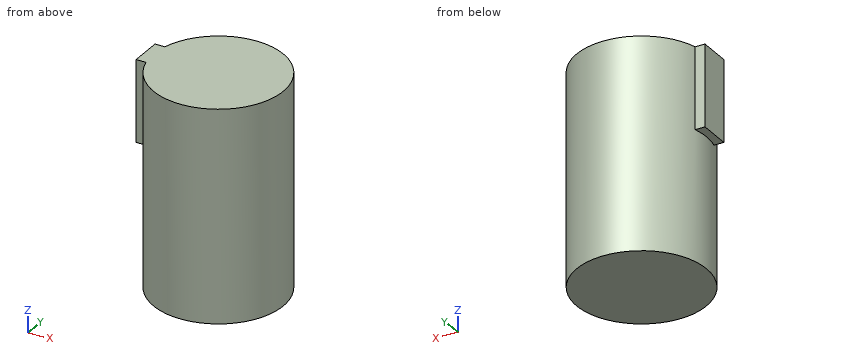
```python
from build123d import *

# Parameters (mm, degrees)
BOSS_EXTRUDE1_DEPTH = 25
BOSS_EXTRUDE3_START = 39.8
SKETCH2_R           = 19.9
BOSS_EXTRUDE3_DEPTH = 39.8


with BuildPart() as part:
    # Sketch1 → Boss-Extrude1 (new body)
    with BuildSketch(Plane(origin=(0, 0, 0), x_dir=(0, 1, 0), z_dir=(0, 0, 1))):
        with BuildLine():
            Line((-4.9, 22.3), (4.9, 22.3))
            Line((4.9, 22.3), (4.9, 19.287301522))
            ThreePointArc((4.9, 19.287301522), (0, -19.9), (-4.9, 19.287301522))
            Line((-4.9, 19.287301522), (-4.9, 22.3))
        make_face()
    extrude(amount=BOSS_EXTRUDE1_DEPTH)

    # Sketch2 → Boss-Extrude3 (add)
    with BuildSketch(Plane(origin=(0, 0, 0), x_dir=(1, 0, 0), z_dir=(0, 0, -1)).offset(BOSS_EXTRUDE3_START)):
        with Locations(Location((0, 0, 0), (0, 0, 180))):
            Circle(SKETCH2_R)
    extrude(amount=-BOSS_EXTRUDE3_DEPTH)


solid = part.part
```
Read the model definition and answer for the solid it produces. Units are mm, in the model's axes. Give positions to 0.01 mm unless a question says otherwise; leave off trailing zeros. Loops run counter-clockwise (first coordinate to the right, second up) from the corner with the lowest first, then second, coordinate; pieces in that order, holes last.
Item 1: The part is cut by section A-A (y = 0). Write down the section's boundary in (x, z), and give its area (3 significant figures).
Item 2: The part is cut by section C-C (x = 17). Write down the section's boundary in (y, z).
Item 3: The part is cut by section B-B (z = 4.5). Write down the section's boundary in (x, y).
Item 4: Find the intervals of material crossed by line 1 along X through (y, z) = (0.5, -11); line 2 along Y through (x, z) = (-20, 0.5); line 3 along X through (y, z) = (18, 6), in increasing order.
Item 5: The part is cut by section D-D (z = -21). Write down the section's boundary in (x, y).
Item 6: Each of these flat-tipped pins is pushed along its axis until it touches: pin 1 Ø2 at (x, z) = (5, 18) entering from +Y; pin 2 Ø0.9 at (x, z) = (-21, 14.5) entering from -Y; pin 3 Ø3 at (y, z) = (-3, 3) entering from +X. Where does it stop, or does it pass through?
Taken from the geometry:
1. outline: (-22.3, 0) - (-19.9, 0) - (-19.9, -39.8) - (19.9, -39.8) - (19.9, 25) - (-22.3, 25) - close
1. area: 2,640 mm2
2. outline: (-10.34, -39.8) - (10.34, -39.8) - (10.34, 25) - (-10.34, 25) - close
3. outline: (-22.3, -4.9) - (-19.29, -4.9) arc R19.9 ccw (long way) to (-19.29, 4.9) - (-22.3, 4.9) - close
4. line 1: x = -19.89 to 19.89
4. line 2: y = -4.9 to 4.9
4. line 3: x = -8.49 to 8.49
5. outline: circle Ø39.8 at (0, 0)
6. pin 1: stops at y = 19.49
6. pin 2: stops at y = -4.9
6. pin 3: stops at x = 19.84
